from build123d import *

# Parameters (mm, degrees)
LED_BASE_BOSS_EXTRUDE1_DEPTH       = 2.4
PIN_RIGHT_BOSS_EXTRUDE2_DEPTH      = 2.2
PIN_RIGHT_SPACE_CUT_EXTRUDE1_REACH = 11.113
SKETCH5_W                          = 3.6
SKETCH5_H                          = 0.7
SKETCH6_R                          = 2.95
HEATSINK_BOSS_EXTRUDE3_DEPTH       = 0.1


with BuildPart() as part:
    # Sketch1 → LED Base Boss-Extrude1 (new body)
    with BuildSketch(Plane(origin=(0, 0, 0), x_dir=(1, 0, 0), z_dir=(0, 1, 0))):
        with BuildLine():
            Line((-3.6, 1.743559577), (-3.6, -1.743559577))
            ThreePointArc((-3.6, -1.743559577), (0, -4), (3.6, -1.743559577))
            Line((3.6, -1.743559577), (3.6, 1.743559577))
            ThreePointArc((3.6, 1.743559577), (0, 4), (-3.6, 1.743559577))
        make_face()
    extrude(amount=LED_BASE_BOSS_EXTRUDE1_DEPTH)

    # Sketch3 → LED Lens Revolve2 (revolve)
    with BuildSketch(Plane.XY):
        with BuildLine():
            Line((2.6, 2.4), (0, 2.4))
            Line((0, 2.4), (0, 5.2))
            ThreePointArc((0, 5.2), (1.910497317, 4.366890366), (2.6, 2.4))
        make_face()
    revolve(axis=Axis((0, 5.2, 0), (0, -1, 0)))

    # Sketch4 → Pin Right Boss-Extrude2 (add, symmetric)
    with BuildSketch(Plane.XY):
        with BuildLine():
            Line((3.6, 1.3), (4.9, 1.3))
            ThreePointArc((4.9, 1.3), (5.182842712, 1.182842712), (5.3, 0.9))
            Line((5.3, 0.9), (5.3, 0.4))
            ThreePointArc((5.3, 0.4), (5.329289322, 0.329289322), (5.4, 0.3))
            Line((5.4, 0.3), (7.2, 0.3))
            Line((7.2, 0.3), (7.2, 0))
            Line((7.2, 0), (5.4, 0))
            ThreePointArc((5.4, 0), (5.117157288, 0.117157288), (5, 0.4))
            Line((5, 0.4), (5, 0.9))
            ThreePointArc((5, 0.9), (4.970710678, 0.970710678), (4.9, 1))
            Line((4.9, 1), (3.6, 1))
            Line((3.6, 1), (3.6, 1.3))
        make_face()
    pin_right_boss_extrude2 = extrude(amount=PIN_RIGHT_BOSS_EXTRUDE2_DEPTH, both=True)

    # Pin Right Space Cut-Extrude1: up to this face of the body (flat: up to its plane)
    pin_right_space_cut_extrude1_end = Plane(part.part.faces().sort_by_distance((6.3, 0, 0))[0])
    # Sketch5 → Pin Right Space Cut-Extrude1 (cut, up to the picked face)
    with BuildSketch(Plane(origin=(0, 1.3, 0), x_dir=(1, 0, 0), z_dir=(0, 1, 0)), mode=Mode.PRIVATE) as pin_right_space_cut_extrude1_sk1:
        with Locations((5.4, 0.85)):
            Rectangle(SKETCH5_W, SKETCH5_H)
    pin_right_space_cut_extrude1_tool1 = split(extrude(pin_right_space_cut_extrude1_sk1.sketch, amount=-PIN_RIGHT_SPACE_CUT_EXTRUDE1_REACH, mode=Mode.PRIVATE), bisect_by=pin_right_space_cut_extrude1_end, keep=Keep.BOTH, mode=Mode.PRIVATE)
    # Sketch5 → Pin Right Space Cut-Extrude1 (cut, up to the picked face)
    with BuildSketch(Plane(origin=(0, 1.3, 0), x_dir=(1, 0, 0), z_dir=(0, 1, 0)), mode=Mode.PRIVATE) as pin_right_space_cut_extrude1_sk2:
        with Locations((5.4, -0.85)):
            Rectangle(SKETCH5_W, SKETCH5_H)
    pin_right_space_cut_extrude1_tool2 = split(extrude(pin_right_space_cut_extrude1_sk2.sketch, amount=-PIN_RIGHT_SPACE_CUT_EXTRUDE1_REACH, mode=Mode.PRIVATE), bisect_by=pin_right_space_cut_extrude1_end, keep=Keep.BOTH, mode=Mode.PRIVATE)
    pin_right_space_cut_extrude1_1 = pin_right_space_cut_extrude1_tool1.solids().sort_by(Axis((5.4, 1.3, -0.85), (0, -1, 0)))[0]
    add(pin_right_space_cut_extrude1_1, mode=Mode.SUBTRACT)
    pin_right_space_cut_extrude1_2 = pin_right_space_cut_extrude1_tool2.solids().sort_by(Axis((5.4, 1.3, 0.85), (0, -1, 0)))[0]
    add(pin_right_space_cut_extrude1_2, mode=Mode.SUBTRACT)
    pin_right_space_cut_extrude1 = pin_right_space_cut_extrude1_1 + pin_right_space_cut_extrude1_2  # Pin Right Space Cut-Extrude1 as one shape, for the pattern or mirror that repeats it

    # Pin Left Mirror1: Pin Right Boss-Extrude2, Pin Right Space Cut-Extrude1 across plane
    add(pin_right_boss_extrude2.mirror(Plane(origin=(0, 0, 0), x_dir=(0, 0, 1), z_dir=(1, 0, 0))))
    add(pin_right_space_cut_extrude1.mirror(Plane(origin=(0, 0, 0), x_dir=(0, 0, 1), z_dir=(1, 0, 0))), mode=Mode.SUBTRACT)

    # Sketch6 → Heatsink Boss-Extrude3 (add)
    with BuildSketch(Plane.XZ):
        with Locations(Location((0, 0, 0), (0, 0, 90))):
            Circle(SKETCH6_R)
    extrude(amount=HEATSINK_BOSS_EXTRUDE3_DEPTH)


solid = part.part
Design review of the part built by this model. Coordinates are the model's own, in mm. A direction names the side the tool comes from. Round coordinates to 2 decimals unless told otherwise and drop trailing zeros. Order: outer loops, then holes, each group sorted by start corner. A loop starts at its lowest first (then second) coordinate and runs counter-clockwise, first axis right, second up.
1) Consider section D-D (x = 1.5). State the section outline as (y, z) points.
The answers:
outline: (-0.1, -2.54) - (0, -2.54) - (0, -3.71) - (2.4, -3.71) - (2.4, -2.12) arc R2.13 ccw (long way) to (2.4, 2.12) - (2.4, 3.71) - (0, 3.71) - (0, 2.54) - (-0.1, 2.54) - close
2) Consider section B-B (x = 0). State the section outline as (y, z) points, plus the area to 3 significant figures.
The answers:
outline: (-0.1, -2.95) - (0, -2.95) - (0, -4) - (2.4, -4) - (2.4, -2.6) arc R2.61 ccw (long way) to (2.4, 2.6) - (2.4, 4) - (0, 4) - (0, 2.95) - (-0.1, 2.95) - close
area: 31.5 mm2
3) Clearance check with flat-ended pins moving along their axes: pin 1 Ø0.8 at (x, z) = (4.5, -2) entering from +Y; pin 2 Ø0.6 at (x, y) = (6, 0.5) entering from -Z; pin 3 Ø1.1 at (x, z) = (-4, 0) entering from +Y. State where each tip first meets the part, or that it passes through.
The answers:
pin 1: stops at y = 1.3
pin 2: stops at z = -2.2
pin 3: stops at y = 2.4
4) Machinability: for faces 1 (the flat face through (-6, 0, 0)), 2 (the flat face through (-2, 0, -3)), 3 (the flat face through (4, 1.3, 2)), which of the approach directions +Z, -Z, +X, -X, +Y, -Y give a long, thin tool a straight path to every point of the face, cutting with its end or side? Answer none if there is none.
The answers:
face 1: +Z, -Z, -X, -Y
face 2: -Y
face 3: +Z, -Z, +X, +Y
5) For L1, parallel to X at y = 0.85, z = 1.5; L2, parallel to Y at x = -2, z = 3; L3, parallel to Y at x = -6, z = -1.5, list the stretches that pass through material, from the lowest coordinate up.
The answers:
L1: x = -5.3 to -5, -3.6 to 3.6, 5 to 5.3
L2: y = 0 to 2.4
L3: y = 0 to 0.3
6) Consider section C-C (y = 1.7). State the section outline as (x, z) points, plus the area to 3 significant figures.
The answers:
outline: (-3.6, -1.74) arc R4 ccw to (3.6, -1.74) - (3.6, 1.74) arc R4 ccw to (-3.6, 1.74) - close
area: 48.4 mm2
7) Draft analysis for pull direction X (two halves, no side actions). For faces 4 (the flat face through (4, 1, -2)), 5 (the flat face through (4, 1.3, -2)), 6 (the flat face through (-4, 1, 0)), state which applies: released by +X, released by -X, zero draft, split by the parting line, or undercut.
The answers:
face 4: undercut
face 5: zero draft
face 6: undercut
